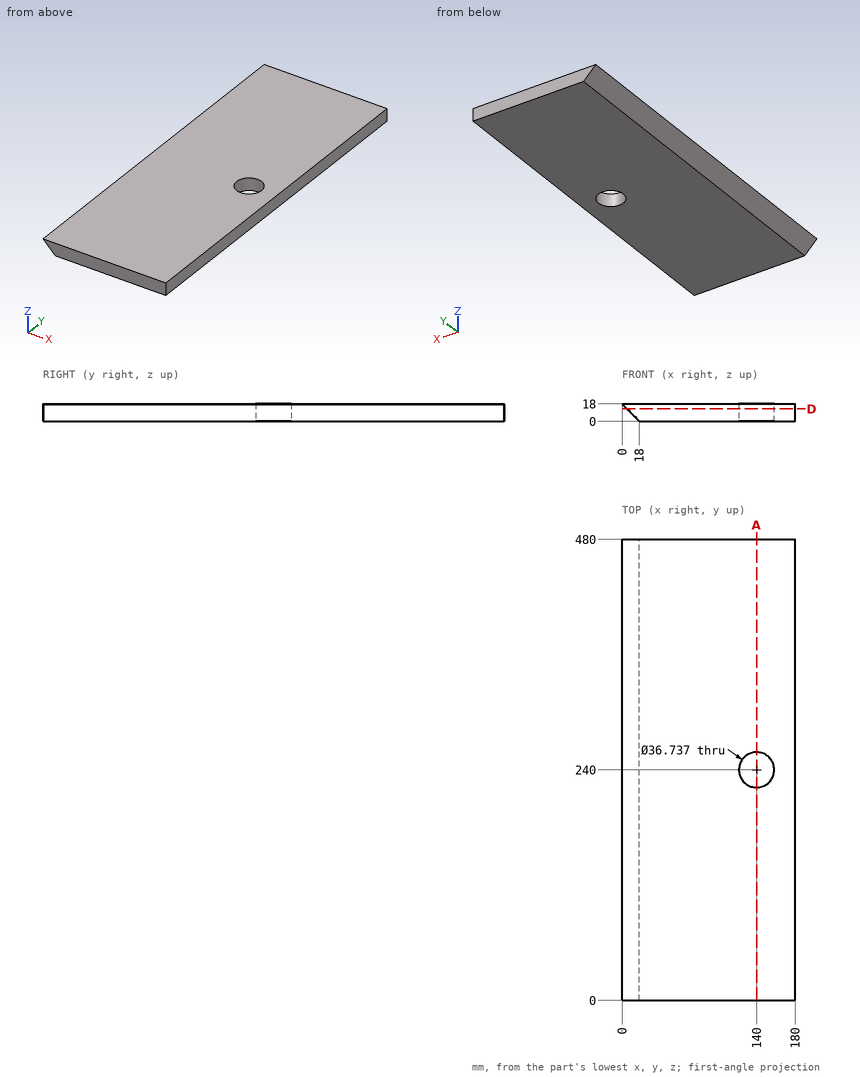
Part print with two shaded views. Sizes in mm from the minimum x, y, z corner. Round coordinates to 2 decimals unless told otherwise and drop trailing zeros. Loops run counter-clockwise (first coordinate to the right, second up) from the corner with the lowest first, then second, coordinate; pieces in that order, holes last. Notation, with made-up numbers: M 30.5,-30 L 60.5,-30 A15 cw 60.5,-17 Z; hole C -6.75,4 d10. An arc over 180 degrees is marked long. Return JSON: item names as keys, results as strings. Group by question number.
(1) Saw through at A-A, the plane x = 140. List the corners of the cut face in (y, z).
(2) Drop flat-ended pins along their axis: P1, Ø1, axis at y = 329.5, z = 6.5, coming from the -X side; P2, Ø2, axis at y = 341.5, z = 10, coming from the -X side; P3, Ø2, axis at y = 143, z = 7.5, coming from the -X side. Give the stop position or say it passes through.
(3) Saw through at D-D, the plane z = 13. List the corners of the cut face in (x, y).
(4) Wall check: probe 1 along Y at (x, z) = (140, 6.5); probe 2 along Y at (x, z) = (146, 16); probe 3 along X at (y, z) = (252.5, 1). Give the ranges that are in metal, low to high. Write a range as [from, to].
Answer list:
{
 "1": {"outline": "M 0,0 L 221.63,0 L 221.63,18 L 0,18 Z; M 258.37,0 L 480,0 L 480,18 L 258.37,18 Z"},
 "2": {"P1": "x = 11", "P2": "x = 7", "P3": "x = 9.5"},
 "3": {"outline": "M 5,0 L 180,0 L 180,480 L 5,480 Z; hole C 140,240 d36.74"},
 "4": {"probe 1": "[0, 221.63], [258.37, 480]", "probe 2": "[0, 222.64], [257.36, 480]", "probe 3": "[17, 126.54], [153.46, 180]"}
}
